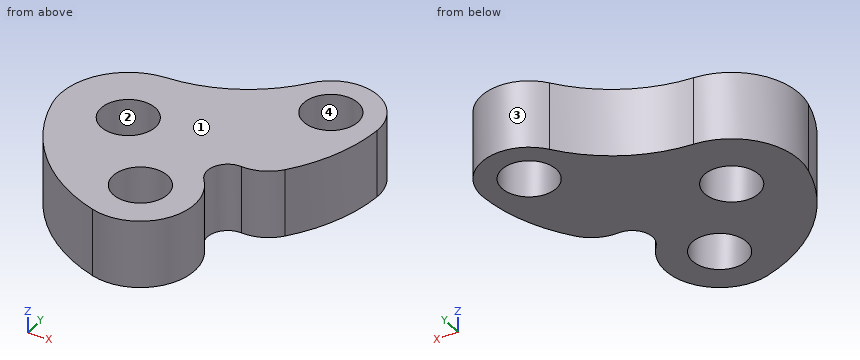
```python
from build123d import *

# Parameters (mm, degrees)
F0_R     = 10
F1_DEPTH = 25


with BuildPart() as f1:
    # F0 (on Top) → F1 (new body)
    with BuildSketch(Plane.XY):
        with BuildLine():
            ThreePointArc((-10.5878, -49.155795), (11.831524, -41.050494), (10.566127, -17.244596))
            ThreePointArc((10.566127, -17.244596), (9.652404, -9.071889), (16.782416, -4.974213))
            ThreePointArc((16.782416, -4.974213), (23.692785, -3.734072), (29.28189, 0.514817))
            ThreePointArc((29.28189, 0.514817), (38.506241, 16.164452), (42.624255, 33.857436))
            ThreePointArc((42.624255, 33.857436), (31.349021, 51.369659), (11.30918, 45.693954))
            ThreePointArc((11.30918, 45.693954), (-6.314116, 30.95087), (-28.499794, 24.973009))
            ThreePointArc((-28.499794, 24.973009), (-47.356712, 14.975562), (-51.623254, -5.93685))
            ThreePointArc((-51.623254, -5.93685), (-36.850918, -33.001447), (-10.5878, -49.155795))
        make_face()
        with Locations((-27.338407, 0)):
            Circle(F0_R, mode=Mode.SUBTRACT)
        with Locations((-4.838407, -30)):
            Circle(F0_R, mode=Mode.SUBTRACT)
        with Locations((25.161593, 35)):
            Circle(F0_R, mode=Mode.SUBTRACT)
    extrude(amount=F1_DEPTH)


solid = f1.part
```
Can you work these out from the model? Positions are in its coordinate system, mm. Face numbers are marked on the shaded views. Coordinates: 2 decimals unless noted, no trailing zeros. Loops run counter-clockwise (first coordinate to the right, second up) from the corner with the lowest first, then second, coordinate; pieces in that order, holes last.
1) For pin 1 (5 mm diameter, centred on x = -27, z = 12.5, fed in from +Y); pin 2 (3 mm diameter, centred on y = 3, z = 4.5, fed in from +X); pin 3 (2 mm diameter, centred on x = 17, z = 16, fed in from +Y), each with a flat end and sliding along its axis, tell me the tip position at first contact or that it passes through.
2) Imagine slicing it at C-C on z = 6.5. List the corners of the cut face in (x, y) for me, plus the area to 3 significant figures.
3) Thinking about a two-plate mould opening in X: for the marked faces 1, 2, 3 and 4, which applies, pulls with the +X half, pulls with the -X half, needs draft (parallel to the pull), parting line crosses it, or undercut?
4) I need wall thicknesses on probe 1 along Y at (x, z) = (-29, 18.5); probe 2 along X at (y, z) = (34, 20); probe 3 along Y at (x, z) = (-25.5, 18.5). Which ranges of each line are inside material? Lowest first, please.
5) Imagine slicing it at A-A on y = -30. List the corners of the cut face in (x, z) for me.
6) Imagine slicing it at B-B on x = 32.5. List the corners of the cut face in (y, z) for me.
7) Imagine slicing it at D-D on y = 22. List the corners of the cut face in (x, z) for me, plus the area to 3 significant figures.
Completed:
1. pin 1: stops at y = 25.31
1. pin 2: stops at x = 32.27
1. pin 3: stops at y = 50.97
2. outline: (-51.62, -5.94) arc R60 ccw to (-10.59, -49.16) arc R20 ccw to (10.57, -17.24) arc R7.5 cw to (16.78, -4.97) arc R15 ccw to (29.28, 0.51) arc R60 ccw to (42.62, 33.86) arc R17.5 ccw to (11.31, 45.69) arc R53.43 cw to (-28.5, 24.97) arc R25 ccw to start; hole circle Ø20 at (-27.34, 0); hole circle Ø20 at (-4.84, -30); hole circle Ø20 at (25.16, 35)
2. area: 4,790 mm2
3. face 1: needs draft
3. face 2: undercut
3. face 3: parting line crosses it
3. face 4: undercut
4. probe 1: y = -39.94 to -9.86, 9.86 to 24.94
4. probe 2: x = -1.18 to 15.21, 35.11 to 42.63
4. probe 3: y = -42.34 to -9.83, 9.83 to 25.2
5. outline: (-39.52, 0) - (-14.84, 0) - (-14.84, 25) - (-39.52, 25) - close; (5.16, 0) - (15.16, 0) - (15.16, 25) - (5.16, 25) - close
6. outline: (4.84, 0) - (28.21, 0) - (28.21, 25) - (4.84, 25) - close; (41.79, 0) - (50.89, 0) - (50.89, 25) - (41.79, 25) - close
7. outline: (-39.21, 0) - (40.5, 0) - (40.5, 25) - (-39.21, 25) - close
7. area: 1,990 mm2
